```python
from build123d import *

# Parameters (mm, degrees)
F0_R     = 1.5875
F1_DEPTH = 25.4
F2_R     = 3.175
F2_R_2   = 1.5875
F3_DEPTH = 2.54
F4_R     = 2.53999
F5_SIZE2 = 5.08
F5_SIZE  = 1.27


# Not quite as in the source:
# - a fillet or chamfer is up to 0.001 mm smaller than in the source, because OpenCascade refuses the exact size


with BuildPart() as f1:
    # F0 (on Right) → F1 (new body)
    with BuildSketch(Plane.YZ):
        Circle(F0_R)
    extrude(amount=-F1_DEPTH)

    # F2 (on face) → F3 (join)
    with BuildSketch(Plane(origin=(-25.4, 0, 0), x_dir=(0, -1, 0), z_dir=(-1, 0, 0))):
        Circle(F2_R)
        Circle(F2_R_2, mode=Mode.SUBTRACT)
        Circle(F2_R_2)
    extrude(amount=F3_DEPTH)

    # F4 (radius 2.54 in the source; OpenCascade refuses exactly that, so slightly less here)
    f4_edges = [f1.edges().sort_by_distance(p)[0] for p in [
        (-27.94, 3.175, 0),
    ]]
    fillet(f4_edges, radius=F4_R)

    # F5
    f5_edges = [f1.edges().sort_by_distance(p)[0] for p in [
        (0, -1.5875, 0),
    ]]
    f5_side = f1.faces().sort_by_distance((0, 0, 0))[0]
    chamfer(f5_edges, length=F5_SIZE, length2=F5_SIZE2, reference=f5_side)


solid = f1.part
```
The model under review builds one solid part; all positions refer to its coordinate system, in mm. A direction names the side the tool comes from. Round coordinates to 2 decimals unless told otherwise and drop trailing zeros. Order: outer loops, then holes, each group sorted by start corner. A loop starts at its lowest first (then second) coordinate and runs counter-clockwise, first axis right, second up. Notation, with made-up numbers: (81, -30) -> (86, -30) arc R20 cw to (86, 4) -> close; hole circle Ø8 at (-5, 10.25). An arc over 180 degrees is marked (long way). One line per item, written item: value. Start each with the question number.
Q1. Wall thickness on line 1 (Z direction, x = -19.75, y = 0); line 2 (Z direction, x = -20.75, y = 1); line 3 (Y direction, x = -23.5, z = -0.25): over which ranges is each line inside the solid? List them lowest first.
Q2. Machinability: for faces 1 (the face through (-15.1, -0.34, -1.55)), 2 (the face through (-27.94, 0, 0)), which of the approach directions +Z, -Z, +X, -X, +Y, -Y give a long, thin tool a straight path to every point of the face, cutting with its end or side? Answer none if there is none.
Q3. Take a section at A-A (x = -23.75). Write out the cut boundary in (y, z) (1 decimal).
Q4. Clearance check with flat-ended pins moving along their axes: pin 1 Ø1 at (x, z) = (-6.5, 2.5) entering from -Y; pin 2 Ø3 at (x, z) = (-3, 1) entering from -Y. State where each tip first meets the part, or that it passes through.
Reported:
1. line 1: z = -1.59 to 1.59
1. line 2: z = -1.23 to 1.23
1. line 3: y = -1.57 to 1.57
2. face 1: +X
2. face 2: +Z, -Z, -X, +Y, -Y
3. outline: circle Ø3.2 at (0, 0)
4. pin 1: passes through
4. pin 2: stops at y = -1.37
